Here's how the part is built. I have some questions about the finished solid (model axes, mm). A direction names the side the tool comes from. Give positions to 0.01 mm unless a question says otherwise; leave off trailing zeros. Order: outer loops, then holes, each group sorted by start corner. A loop starts at its lowest first (then second) coordinate and runs counter-clockwise, first axis right, second up. Notation, with made-up numbers: M 8.5,47 L 21.5,47 A11 cw 21.5,61 Z; hole C 85.25,-22.75 d1. An arc over 180 degrees is marked long. Use one line per item in the form item = value.
from build123d import *

# Parameters (mm, degrees)
SKETCH1_R           = 17.71
BOSS_EXTRUDE1_DEPTH = 2
SKETCH1_3_R         = 16.61
SKETCH1_3_R_2       = 15.81
BOSS_EXTRUDE2_DEPTH = 5
FILLET1_R           = 2
SKETCH3_W           = 7.599801802
SKETCH3_H           = 7.043482716
CUT_EXTRUDE1_DEPTH  = 4.8
FILLET2_R           = 2


# Some blends are built 0.0001 mm under size
with BuildPart() as part:
    # Sketch1 → Boss-Extrude1 (new body)
    with BuildSketch(Plane(origin=(0, 0, 0), x_dir=(1, 0, 0), z_dir=(0, 1, 0))):
        with Locations(Location((0, 0, 0), (0, 0, 270))):
            Circle(SKETCH1_R)
    extrude(amount=BOSS_EXTRUDE1_DEPTH)

    # Sketch1<3> → Boss-Extrude2 (add)
    with BuildSketch(Plane(origin=(0, 0, 0), x_dir=(1, 0, 0), z_dir=(0, 1, 0))):
        with Locations(Location((0, 0, 0), (0, 0, 270))):
            Circle(SKETCH1_3_R)
        with Locations(Location((0, 0, 0), (0, 0, 270))):
            Circle(SKETCH1_3_R_2, mode=Mode.SUBTRACT)
    extrude(amount=BOSS_EXTRUDE2_DEPTH)

    # Fillet1
    fillet1_edges = [part.edges().sort_by_distance(p)[0] for p in [
        (0, 0, -17.71),
    ]]
    fillet(fillet1_edges, radius=FILLET1_R - 0.0001)  # a hair under: the kernel refuses the full size

    # Sketch3 → Cut-Extrude1 (cut)
    with BuildSketch(Plane.XY.offset(20)):
        with Locations((0, 4.688271449)):
            Rectangle(SKETCH3_W, SKETCH3_H)
    extrude(amount=-CUT_EXTRUDE1_DEPTH, mode=Mode.SUBTRACT)

    # Fillet2
    # the kernel refuses this fillet: 2 mm, written as the material it takes off along each edge
    with BuildSketch(Plane(origin=(3.799900901, 2, 15.2), x_dir=(0, 0, -1), z_dir=(-1, 0, 0))) as fillet2_piece_1:
        with BuildLine():
            CenterArc((1.624563802, 2), FILLET2_R, 215.680517758, 54.319482242)
            Line((0, 0.833469909), (-0.032491276, 0.810139307))
            ThreePointArc((-0.032491276, 0.810139307), (-0.04, 0.416734955), (-0.04, 0))
            Line((-0.04, 0), (0, -0.04))
            Line((0, -0.04), (1.624563802, -0.04))
            Line((1.624563802, -0.04), (1.624563802, 0))
        make_face()
    extrude(amount=7.599801803, mode=Mode.SUBTRACT)


solid = part.part
Q1. Thinking about a two-plate mould opening in X: for faces 1 (the face through (0.677, 3.479, -16.596)), 2 (the face through (0, 2, 0)), 3 (the face through (0, 0, 0)), which applies, +X half, -X half, draft (parallel to the pull), parting line (faces both ways), or undercut?
Found:
face_1 = parting line
face_2 = undercut
face_3 = draft
Q2. I want a section at C-C on y = 3.6. Write out the boundary of the cut face in (x, z), then the cut area to 3 significant figures.
Found:
outline = M -3.8,15.35 L -3.8,16.17 A16.61 ccw long 3.8,16.17 L 3.8,15.35 A15.81 cw long Z
area = 75.3 mm²
Q3. I need wall thicknesses on L1, parallel to X at y = 4, z = 0; L2, parallel to Y at x = 5, z = -10.5; L3, parallel to X at y = 3.4, z = 5. Which ranges of each line are inside material? Lowest first, please.
Found:
L1 = -16.61 to -15.81, 15.81 to 16.61
L2 = 0 to 2
L3 = -15.84 to -15, 15 to 15.84
Q4. On a 3-axis mill with a long thin cutter (end or side, diameter ignored), from which of +Z, -Z, +X, -X, +Y, -Y can I reach the whole of each face in a straight line? I mean faces 4 (the face through (-5, 2, -16)), 5 (the face through (3.8, 3, 16)), 6 (the face through (0, 5, -16)). Say none if no direction works.
Found:
face_4 = +Y
face_5 = +Z, +Y
face_6 = +Z, -Z, +X, -X, +Y
Q5. I'm going to push flat-ended pins straight in: pin 1 Ø10 at (x, z) = (-2, -11) entering from +Y; pin 2 Ø1 at (x, y) = (8, 3) entering from +Z; pin 3 Ø9.5 at (x, z) = (-6, -2) entering from +Y; pin 4 Ø2.5 at (x, z) = (1.5, 16) entering from +Y. Where does each tip first touch, or does it pass through?
Found:
pin_1 = 5
pin_2 = 14.82
pin_3 = 2
pin_4 = 1.62
